Autodesk Inventor part; units mm, degrees
ref_plane "Start Plane" through (0, 0, 10) normal (0, 0, 1) x (1, 0, 0)
ref_plane "End Plane" through (0, 0, 100) normal (0, 0, 1) x (1, 0, 0)
ref_plane "Work Plane4" through (0, 0, 10) normal (0, 0, -1) x (-1, 0, 0)
ref_plane "Start Plane" through (0, 0, 10) normal (0, 0, 1) x (1, 0, 0)
ref_plane "End Plane" through (0, 0, 100) normal (0, 0, 1) x (1, 0, 0)
sketch "Sketch" plane through (0, 0, 0) normal (0, 0, 1) x (1, 0, 0)
  line L0 (-10, -7) -> (-10, 7)
  line L1 (-7, 10) -> (7, 10)
  line L2 (10, 7) -> (10, -7)
  line L3 (7, -10) -> (-7, -10)
  arc A0 (-10, -7) -> (-7, -10) centre (-7, -7) ccw
  arc A1 (-7, 10) -> (-10, 7) centre (-7, 7) ccw
  arc A2 (10, 7) -> (7, 10) centre (7, 7) ccw
  arc A3 (7, -10) -> (10, -7) centre (7, -7) ccw
  arc A4 (-7, 8) -> (-8, 7) centre (-7, 7) ccw
  line L4 (-7, 8) -> (7, 8)
  arc A5 (8, 7) -> (7, 8) centre (7, 7) ccw
  line L5 (8, 7) -> (8, -7)
  arc A6 (7, -8) -> (8, -7) centre (7, -7) ccw
  line L6 (7, -8) -> (-7, -8)
  arc A7 (-8, -7) -> (-7, -8) centre (-7, -7) ccw
  line L7 (-8, -7) -> (-8, 7)
  line L8 (0, 14.8698) -> (0, -14.8698) construction
  line L9 (-14.8698, 0) -> (14.8698, 0) construction
  dimension "d7" = 3
  dimension "d10" = 20
  dimension "d11" = 20
  dimension "d12" = 2
  dimension "d15" = 10
  dimension "d16" = 10
extrude "Body" add sketch "Sketch" along normal up to surface (90 mm away) from surface at 10
sketch "Sketch3" plane through (0, 0, 0) normal (0, 0, 1) x (1, 0, 0)
  line L0 (0, 0) -> (10, 0)
ref_plane "Work Plane3" through (0, 0, 0) normal (0, -1, 0) x (1, 0, 0)
sketch "Sketch4" plane through (0, 0, 0) normal (0, -1, 0) x (1, 0, 0)
  line L0 (-2, 10) -> (12, 10)
  line L1 (-2, 100) -> (12, 100)
  dimension "d18" = 90
ref_plane "Work Plane4" through (0, 0, 10) normal (0, 0, -1) x (-1, 0, 0)
split "Split1" plane through (0, 0, 10) removes the side toward (0, 0, -1)
ref_plane "Work Plane5" through (0, 0, 100) normal (0, 0, 1) x (1, 0, 0)
split "Split2" plane through (0, 0, 100) removes the side toward (0, 0, 1)
equation "\"d7\" = G_IR"
equation "\"d10\" = G_H"
equation "\"d11\" = G_W"
equation "\"d12\" = G_T"
equation "\"d15\" = 0.5 * d10"
equation "\"d16\" = 0.5 * d11"
equation "\"d3\" = G_L"
equation "\"G_W\" = 20"
equation "\"G_H\" = 20"
equation "\"G_T\" = 2"
equation "\"G_IR\" = 3"
equation "\"G_L\" = d18"
properties part number "ISO 12633-2 - 20x20x2 - 90" material "Steel, Mild"
Source: CAD feature listing. Evaluate the final solid. Frame: model axes, mm. A direction names the side the tool comes from. Round coordinates to 2 decimals unless told otherwise and drop trailing zeros. Write each loop counter-clockwise with the first axis right and the second up, starting at its lowest first coordinate (ties: lowest second). Pieces come first, ordered by that corner, then holes. Notation, with made-up numbers: M 83.25,-22 L 130.25,-22 A18 ccw 130.25,-4 Z; hole C -10,-10 d3. An arc over 180 degrees is marked long. One line per item, written item: value. Start each with the question number.
Item 1: Set-up query: faces 5 (the cylindrical face through (-9.1, -9.14, 54.37)), 6 (the flat face through (-8, 0, 54)). Return all of +Z, -Z, +X, -X, +Y, -Y with unobstructed straight access to the full face (end or side cutting, diameter ignored); none if empty.
Item 2: Section query A-A (x = -2.5). Return the cut outline in (y, z), plus the area to 3 significant figures.
Item 3: Ray query, L1, parallel to Y at x = 5.5, z = 92; L2, parallel to X at y = -7.75, z = 93.5. Return the intervals inside material, ascending. Write a range as from..to.
Item 4: Mould query, pull axis X, two halves, no side actions, for faces 1 (the flat face through (0, -8, 54)), 2 (the flat face through (-10, 0, 54)), 3 (the flat face through (8, 0, 54)), 4 (the flat face through (0, -10, 54)). Classes: pulls with the +X half, pulls with the -X half, needs draft (parallel to the pull), parting line crosses it, or undercut.
Item 5: Section query C-C (z = 20). Return the cut outline in (x, y).
Result set:
1. face 5: +Z, -Z, -X, -Y
1. face 6: +Z, -Z
2. outline: M -10,10 L -8,10 L -8,100 L -10,100 Z; M 8,10 L 10,10 L 10,100 L 8,100 Z
2. area: 360 mm²
3. L1: y = -10..-8, 8..10
3. L2: x = -9.9..-7.66, 7.66..9.9
4. face 1: undercut
4. face 2: pulls with the -X half
4. face 3: undercut
4. face 4: needs draft
5. outline: M -10,-7 A3 ccw -7,-10 L 7,-10 A3 ccw 10,-7 L 10,7 A3 ccw 7,10 L -7,10 A3 ccw -10,7 Z; hole M -8,-7 A1 ccw -7,-8 L 7,-8 A1 ccw 8,-7 L 8,7 A1 ccw 7,8 L -7,8 A1 ccw -8,7 Z
